Autodesk Inventor part; units mm, degrees
ref_plane "YZ Plane" through (0, 0, 0) normal (1, 0, 0) x (0, 1, 0)
ref_plane "XZ Plane" through (0, 0, 0) normal (0, 1, 0) x (-1, 0, 0)
ref_plane "XY Plane" through (0, 0, 0) normal (0, 0, 1) x (1, 0, 0)
sketch "Sketch1" plane through (0, 0, 0) normal (0, 0, 1) x (1, 0, 0)
  line L0 (0, 0) -> (50.8, 0)
  line L1 (50.8, 0) -> (50.8, 50.8)
  line L2 (50.8, 50.8) -> (0, 50.8)
  line L3 (0, 50.8) -> (0, 0)
  dimension "d0" = 50.8
  dimension "d1" = 50.8
extrude "Extrusion1" add sketch "Sketch1" along normal blind 6.35
sketch "Sketch2" plane through (0, 50.8, 0) normal (0, 1, 0) x (1, 0, 0)
  line L0 (0, 0) -> (50.8, 0)
  line L1 (0, -6.35) -> (50.8, -6.35)
  line L2 (20.3299, 0) -> (30.4899, 0)
  line L3 (30.4899, 0) -> (30.4899, -6.35)
  line L4 (30.4899, -6.35) -> (20.3299, -6.35)
  line L5 (20.3299, -6.35) -> (20.3299, 0)
  dimension "d4" = 10.16
extrude "Extrusion2" cut sketch "Sketch2" against normal blind 10.16
sketch "Sketch3" plane through (50.8, 0, 0) normal (1, 0, 0) x (0, 0, -1)
  line L0 (0, 0) -> (-6.35, 0)
  line L1 (0, 0) -> (-133.35, 0)
  line L2 (-133.35, 0) -> (-133.35, 50.8)
  line L3 (-133.35, 50.8) -> (0, 50.8)
  line L4 (0, 50.8) -> (0, 0)
  dimension "d7" = 133.35
extrude "Extrusion3" add sketch "Sketch3" along normal blind 6.35
sketch "Sketch4" plane through (0, 0, 0) normal (-1, 0, 0) x (0, 0, 1)
  line L0 (133.35, 0) -> (133.35, 50.8)
  line L1 (0, 0) -> (133.35, 0)
  line L2 (133.35, 0) -> (133.35, 50.8)
  line L3 (133.35, 50.8) -> (0, 50.8)
  line L4 (0, 50.8) -> (0, 0)
extrude "Extrusion4" add sketch "Sketch4" along normal blind 6.35
sketch "Sketch5" plane through (0, 0, 0) normal (1, 0, 0) x (0, 0, -1)
  line L0 (-6.35, 0) -> (-133.35, 0)
  line L1 (-133.35, 50.8) -> (-6.35, 50.8)
  line L2 (-133.35, 0) -> (-127, 0)
  line L3 (-127, 0) -> (-127, 50.8)
  line L4 (-127, 50.8) -> (-133.35, 50.8)
  line L5 (-133.35, 50.8) -> (-133.35, 0)
  point P0 (0, 0)
  dimension "d12" = 6.35
extrude "Extrusion5" add sketch "Sketch5" along normal blind 50.8
sketch "Sketch6" plane through (57.15, 0, 0) normal (0, -1, 0) x (1, 0, 0)
  line L0 (-57.15, 6.35) -> (-6.35, 6.35)
  line L1 (-57.15, 127) -> (-57.15, 6.35)
  line L2 (-6.35, 6.35) -> (-57.15, 6.35)
  line L3 (-57.15, 6.35) -> (-57.15, 127)
  line L4 (-57.15, 127) -> (-6.35, 127)
  line L5 (-6.35, 127) -> (-6.35, 6.35)
  point P0 (-57.15, 0)
extrude "Extrusion6" add sketch "Sketch6" against normal blind 6.35
equation "\"d5\" = d4"
properties part number "BatteryHolder"
For this review, take the finished solid that the model builds, in its own axes (mm). A direction names the side the tool comes from. Give positions to 0.01 mm unless a question says otherwise; leave off trailing zeros. Loops run counter-clockwise (first coordinate to the right, second up) from the corner with the lowest first, then second, coordinate; pieces in that order, holes last. Notation, with made-up numbers: M 44.5,17 L 69.5,17 A29 cw 69.5,49 Z; hole C 24,-8.75 d9. An arc over 180 degrees is marked long. One line per item, written item: value. Start each with the question number.
Q1. Add section B-B (x = 26.5). Give the boundary of the cut face in (y, z).
Q2. For L1, parallel to X at y = 47.5, z = 62.5; L2, parallel to Z at x = 45.5, y = 15.5; L3, parallel to Z at x = 28.5, y = 46.5, list the stretches that pass through material, from the lowest coordinate up.
Q3. Draft analysis for pull direction Z (two halves, no side actions). For faces 1 (the face through (25, 28, 127)), 2 (the face through (26, 26, 0)), 3 (the face through (57.15, 26, 68)), state which applies: released by +Z, released by -Z, zero draft, split by the parting line, or undercut.
Q4. Machinability: for faces 4 (the face through (30.49, 46, 3)), 5 (the face through (0, 29, 66)), 6 (the face through (25, 0, 68)), which of the approach directions +Z, -Z, +X, -X, +Y, -Y give a long, thin tool a straight path to every point of the face, cutting with its end or side? Answer none if there is none.
Q5. Add section A-A (y = 46). Give the boundary of the cut face in (x, z).
Q6. Clearance check with flat-ended pins moving along their axes: pin 1 Ø2 at (x, z) = (40.5, 83.5) entering from -Y; pin 2 Ø1.9 at (x, z) = (25, 3) entering from +Y; pin 3 Ø8 at (x, z) = (19, 38) entering from +Y. State where each tip first meets the part, or that it passes through.
Q7. Add section C-C (z = 85.5). Give the boundary of the cut face in (x, y).
Q8. Add section D-D (y = 8.5). Give the boundary of the cut face in (x, z), and give its area (3 significant figures).
Reply:
1. outline: M 0,0 L 40.64,0 L 40.64,6.35 L 6.35,6.35 L 6.35,127 L 50.8,127 L 50.8,133.35 L 0,133.35 Z
2. L1: -6.35 to 0, 50.8 to 57.15
2. L2: 0 to 6.35, 127 to 133.35
2. L3: 127 to 133.35
3. face 1: undercut
3. face 2: released by -Z
3. face 3: zero draft
4. face 4: -Z, +Y
4. face 5: +Y
4. face 6: +Z, -Z, +X, -X, -Y
5. outline: M -6.35,0 L 20.33,0 L 20.33,6.35 L 0,6.35 L 0,127 L 50.8,127 L 50.8,6.35 L 30.49,6.35 L 30.49,0 L 57.15,0 L 57.15,133.35 L -6.35,133.35 Z
6. pin 1: y = 0
6. pin 2: y = 40.64
6. pin 3: y = 6.35
7. outline: M -6.35,0 L 57.15,0 L 57.15,50.8 L 50.8,50.8 L 50.8,6.35 L 0,6.35 L 0,50.8 L -6.35,50.8 Z
8. outline: M -6.35,0 L 57.15,0 L 57.15,133.35 L -6.35,133.35 Z; hole M 0,6.35 L 50.8,6.35 L 50.8,127 L 0,127 Z
8. area: 2,340 mm²
